Part model, mm, in its own coordinate system. A direction names the side the tool comes from. Round coordinates to 2 decimals unless told otherwise and drop trailing zeros. Write each loop counter-clockwise with the first axis right and the second up, starting at its lowest first coordinate (ties: lowest second). Pieces come first, ordered by that corner, then holes.
1) Which spindle directions (+Z, -Z, +X, -X, +Y, -Y) get a long thin tool onto all of the face, cutting with end or side? Do faces 4 (the flat face through (57, 0, 0)), 5 (the cylindrical face through (57.494, -1.426, 29.704)), 6 (the flat face through (-60, 0, 0)), 7 (the cylindrical face through (57.49, -1.5, -29.78)). Say none if no direction does.
2) Flat gauge pins, fed straight in: pin 1 (17.5 mm diameter, centred on x = 61.55, y = -13.14, fed in from +Z); pin 2 (3 mm diameter, centred on y = 10, z = -9, fed in from -X); pin 3 (9 mm diameter, centred on x = -57, z = -2, fed in from +Y); pin 4 (1.5 mm diameter, centred on y = 13.5, z = -3, fed in from +X). Where does each tip first touch, or does it go through?
3) Pull direction Y, two halves, no side cores. Call faces 1 (the flat face through (-74.899, -12, 0)), 2 (the cylindrical face through (-59.959, -1.426, 29.704)), 3 (the cylindrical face through (54.036, -13.47, -0.437)): +Y half, -Y half, draft (parallel to the pull), parting line (faces both ways), or undercut.
4) Saw through at C-C on z = 2. Write the cut outline in (x, y), and give its area (3 significant figures).
5) Saw through at B-B on x = -59. Write the cut outline in (y, z), and give its area (3 significant figures).
6) Saw through at A-A on y = -18. Write the cut outline in (x, z), and give its area (3 significant figures).
7) Drill centre lines: L1, parallel to X at y = -15, z = 24; L2, parallel to X at y = -11, z = -13; L3, parallel to Y at x = 61, z = -18. Where is each one in solid material? Low to high.
8) Saw through at D-D on y = 7.5. Write the cut outline in (x, z).
```python
from build123d import *

# Parameters (mm, degrees)
F0_W         = 149.7976481915
F0_H         = 62.41568923
F1_DEPTH     = 25
F2_W         = 90.8637270331
F2_H         = 62.41568923
F3_DEPTH     = 20
F4_R         = 7.5225312021
F5_DEPTH     = 100
F6_R         = 6.2150283999
F7_DEPTH     = 100
F8_R         = 5
F9_T1_DEPTH  = 24.4669605792
F9_S5_W      = 5
F9_S5_H      = 5
F9_T6_DEPTH  = 5
F9_S11_W     = 5
F9_S11_H     = 5
F9_T12_DEPTH = 5
F10_R        = 5


# Not quite as in the source:
# - a fillet or chamfer that OpenCascade refuses, or shapes differently, is made with other operations: its cross-section is extruded or revolved along the edge and cut away or added


with BuildPart() as f1:
    # F0 (on Front) → F1 (new body)
    with BuildSketch(Plane.XZ):
        Rectangle(F0_W, F0_H)
    extrude(amount=F1_DEPTH)

    # F2 (on face) → F3 (join)
    with BuildSketch(Plane(origin=(0, 0, 0), x_dir=(-1, 0, 0), z_dir=(0, 1, 0))):
        Rectangle(F2_W, F2_H)
    extrude(amount=F3_DEPTH)

    # F4 (on face) → F5 (cut)
    with BuildSketch(Plane(origin=(0, 0, -31.207844615), x_dir=(1, 0, 0), z_dir=(0, 0, -1))):
        with Locations((61.5517050582, 13.1388221845)):
            Circle(F4_R)
    extrude(amount=-F5_DEPTH, mode=Mode.SUBTRACT)

    # F6 (on face) → F7 (cut)
    with BuildSketch(Plane.XY.offset(31.207844615)):
        with Locations((-57.4441173465, -15.3550794757)):
            Circle(F6_R)
    extrude(amount=-F7_DEPTH, mode=Mode.SUBTRACT)

    # F8
    f8_edges = [f1.edges().sort_by_distance(p)[0] for p in [
        (45.431864, 20, 0),
        (-45.431864, 20, 0),
        (74.898824, -12.5, -31.207845),
        (74.898824, -12.5, 31.207845),
        (74.898824, 0, 0),
        (74.898824, -25, 0),
        (0, 20, 31.207845),
        (0, 20, -31.207845),
    ]]
    fillet(f8_edges, radius=F8_R)

    # F9: fillet of radius 5 on 2 edges, made by hand

    # F9_s2 → F9_t1 (cut)
    with BuildSketch(Plane.YZ.offset(45.4318635166)):
        with BuildLine():
            ThreePointArc((-5, -31.207844615), (-1.4644660941, -29.7433785209), (0, -26.207844615))
            Line((0, -26.207844615), (0, -31.207844615))
            Line((0, -31.207844615), (-5, -31.207844615))
        make_face()
        with BuildLine():
            ThreePointArc((0, 26.207844615), (-1.4644660941, 29.7433785209), (-5, 31.207844615))
            Line((-5, 31.207844615), (0, 31.207844615))
            Line((0, 31.207844615), (0, 26.207844615))
        make_face()
    extrude(amount=F9_T1_DEPTH, mode=Mode.SUBTRACT)


with BuildPart() as f9_tool4:
    # F9_s5 → F9_t6 (new body)
    with BuildSketch(Plane.XZ.offset(5)):
        with Locations((72.3988240957, 28.707844615)):
            Rectangle(F9_S5_W, F9_S5_H)
    extrude(amount=-F9_T6_DEPTH)

    # F9_s7 → F9_t8 (revolve, cut)
    with BuildSketch(Plane(origin=(69.8988240957, -5, 26.207844615), x_dir=(-0.7071067812, 0, -0.7071067812), z_dir=(0.7071067812, 0, -0.7071067812))):
        with BuildLine():
            ThreePointArc((0, -5), (5, 0), (0, 5))
            Line((0, 5), (0, -5))
        make_face()
    revolve(axis=Axis((69.8988240957, -5, 26.207844615), (0, 1, 0)), mode=Mode.SUBTRACT)


with BuildPart() as f1_1:
    add(f1.part)

    # F9_t3: cut F9_tool4
    add(f9_tool4.part, mode=Mode.SUBTRACT)


with BuildPart() as f9_tool10:
    # F9_s11 → F9_t12 (new body)
    with BuildSketch(Plane.XY.offset(-26.207844615)):
        with Locations((72.3988240957, -2.5)):
            Rectangle(F9_S11_W, F9_S11_H)
    extrude(amount=-F9_T12_DEPTH)

    # F9_s13 → F9_t14 (revolve, cut)
    with BuildSketch(Plane(origin=(69.8988240957, -5, -26.207844615), x_dir=(-0.7071067812, -0.7071067812, 0), z_dir=(0.7071067812, -0.7071067812, 0))):
        with BuildLine():
            ThreePointArc((0, -5), (5, 0), (0, 5))
            Line((0, 5), (0, -5))
        make_face()
    revolve(axis=Axis((69.8988240957, -5, -26.207844615), (0, 0, -1)), mode=Mode.SUBTRACT)


with BuildPart() as f1_2:
    add(f1_1.part)

    # F9_t9: cut F9_tool10
    add(f9_tool10.part, mode=Mode.SUBTRACT)

    # F10
    f10_edges = [f1_2.edges().sort_by_distance(p)[0] for p in [
        (-60.165344, 0, -31.207845),
        (-60.165344, 0, 31.207845),
    ]]
    fillet(f10_edges, radius=F10_R)


solid = f1_2.part
```
Completed:
1. face 4: +Z, -Z, +X, +Y
1. face 5: +Z, +X, +Y
1. face 6: +Z, -Z, -X, +Y
1. face 7: -Z, +X, +Y
2. pin 1: stops at z = 31.21
2. pin 2: stops at x = -45.43
2. pin 3: stops at y = 0
2. pin 4: stops at x = 45.43
3. face 1: draft
3. face 2: +Y half
3. face 3: undercut
4. outline: (-74.9, -25) - (69.9, -25) arc R5 ccw to (74.9, -20) - (74.9, -5) arc R5 ccw to (69.9, 0) - (45.43, 0) - (45.43, 15) arc R5 ccw to (40.43, 20) - (-40.43, 20) arc R5 ccw to (-45.43, 15) - (-45.43, 0) - (-74.9, 0) - close; hole circle Ø12.43 at (-57.44, -15.36); hole circle Ø15.05 at (61.55, -13.14)
4. area: 5,240 mm2
5. outline: (-25, -31.21) - (-21.37, -31.21) - (-21.37, 31.21) - (-25, 31.21) - close; (-9.34, -31.21) - (-5, -31.21) arc R5 ccw to (0, -26.21) - (0, 26.21) arc R5 ccw to (-5, 31.21) - (-9.34, 31.21) - close
5. area: 799 mm2
6. outline: (-74.9, -31.21) - (-63.07, -31.21) - (-63.07, 31.21) - (-74.9, 31.21) - close; (-51.82, -31.21) - (55.81, -31.21) - (55.81, 31.21) - (-51.82, 31.21) - close; (67.29, -31.21) - (69.9, -31.21) arc R5 ccw to (74.9, -26.21) - (74.9, 26.21) arc R5 ccw to (69.9, 31.21) - (67.29, 31.21) - close
6. area: 7,920 mm2
7. L1: x = -74.9 to -63.65, -51.24 to 54.26, 68.84 to 74.9
7. L2: x = -74.9 to -61.88, -53.01 to 54.34, 68.76 to 74.9
7. L3: y = -25 to -20.64, -5.64 to 0
8. outline: (-45.43, -31.21) - (45.43, -31.21) - (45.43, 31.21) - (-45.43, 31.21) - close
